```python
from build123d import *

# Parameters (mm, degrees)
COLLAR_STOCK_SKETCH_R             = 9
COLLAR_STOCK_DEPTH                = 6
AXLE_COLLAR_BORE_SKETCH_R         = 6.05
AXLE_COLLAR_BORE_DEPTH            = 6.2
POSITIVE_SPRING_PIN_BORE_SKETCH_R = 1.5
POSITIVE_SPRING_PIN_BORE_DEPTH    = 20


with BuildPart() as part:
    # Collar stock sketch → Collar stock (new body)
    with BuildSketch(Plane(origin=(0, -246.5, 0), x_dir=(1, 0, 0), z_dir=(0, 1, 0))):
        with Locations(Location((-19.009182883, 53.244882879, 0), (0, 0, 270))):
            Circle(COLLAR_STOCK_SKETCH_R)
    extrude(amount=COLLAR_STOCK_DEPTH)

    # Axle collar bore sketch → Axle collar bore (cut)
    with BuildSketch(Plane(origin=(0, -246.6, 0), x_dir=(1, 0, 0), z_dir=(0, 1, 0))):
        with Locations(Location((-19.009182883, 53.244882879, 0), (0, 0, 270))):
            Circle(AXLE_COLLAR_BORE_SKETCH_R)
    extrude(amount=AXLE_COLLAR_BORE_DEPTH, mode=Mode.SUBTRACT)

    # Positive spring pin bore sketch → Positive spring pin bore (cut)
    with BuildSketch(Plane(origin=(-29.009182883, 0, 0), x_dir=(0, 0, -1), z_dir=(1, 0, 0))):
        with Locations(Location((53.244882879, -243.5, 0), (0, 0, 180))):
            Circle(POSITIVE_SPRING_PIN_BORE_SKETCH_R)
    extrude(amount=POSITIVE_SPRING_PIN_BORE_DEPTH, mode=Mode.SUBTRACT)


solid = part.part
```
For this review, take the finished solid that the model builds, in its own axes (mm). Give positions to 0.01 mm unless a question says otherwise; leave off trailing zeros. Write each loop counter-clockwise with the first axis right and the second up, starting at its lowest first coordinate (ties: lowest second). Pieces come first, ordered by that corner, then holes. Notation, with made-up numbers: M 22.5,-10 L 59.5,-10 A8 cw 59.5,1 Z; hole C 26.5,31 d10. An arc over 180 degrees is marked long. Answer as a JSON object with one key per item and string values. Group by question number.
Item 1: Consider section B-B on z = -58.75. Write out the cut boundary in (x, y), plus the area to 3 significant figures.
Item 2: Draft analysis for pull direction X (two halves, no side actions). For faces 1 (the cylindrical face through (-27, -243.5, -49.1)), 2 (the cylindrical face through (-17.192, -243.542, -47.474)), 3 (the flat face through (-21, -246.5, -47)), state which applies: +X half, -X half, draft (parallel to the pull), parting line (faces both ways), or undercut.
Item 3: For pin 1 Ø2 at (y, z) = (-243.5, -58.5) entering from -X, flat-tipped, find the tip position at first contact; note if it passes through.
Item 4: Consider section D-D on y = -245.25. Write out the cut boundary in (x, z).
Item 5: For probe 1 along Z at (x, y) = (-16.75, -241.75); probe 2 along Y at (x, z) = (-10.75, -52.5); probe 3 along Z at (x, y) = (-13, -244), list the stretches that pass through material, from the lowest coordinate up. Write a range as [from, to].
Item 6: Consider section A-A on y = -243.5. Write out the cut boundary in (x, z).
Item 7: Consider section C-C on x = -12. Write out the cut boundary in (y, z), plus the area to 3 significant figures.
Check result:
{
 "1": {"outline": "M -26.13,-246.5 L -21.52,-246.5 L -21.52,-240.5 L -26.13,-240.5 Z; M -16.5,-246.5 L -11.89,-246.5 L -11.89,-240.5 L -16.5,-240.5 Z", "area": "55.3 mm^2"},
 "2": {"face 1": "parting line", "face 2": "undercut", "face 3": "draft"},
 "3": {"pin 1": "stops at x = -26.94"},
 "4": {"outline": "C -19.01,-53.24 d18; hole C -19.01,-53.24 d12.1"},
 "5": {"probe 1": "z = [-61.96, -58.86], [-47.63, -44.53]", "probe 2": "y = [-246.5, -244.8], [-242.2, -240.5]", "probe 3": "z = [-59.94, -54.66], [-51.83, -46.54]"},
 "6": {"outline": "M -27.88,-54.74 A9 ccw -10.14,-54.74 L -13.15,-54.74 A6.05 cw -24.87,-54.74 Z; M -27.88,-51.74 L -24.87,-51.74 A6.05 cw -13.15,-51.74 L -10.14,-51.74 A9 ccw Z"},
 "7": {"outline": "M -246.5,-58.89 L -240.5,-58.89 L -240.5,-47.6 L -246.5,-47.6 Z; hole C -243.5,-53.24 d3", "area": "60.7 mm^2"}
}
